Design review of the part built by this model. Coordinates are the model's own, in mm. A direction names the side the tool comes from. Give positions to 0.01 mm unless a question says otherwise; leave off trailing zeros. Write each loop counter-clockwise with the first axis right and the second up, starting at its lowest first coordinate (ties: lowest second). Pieces come first, ordered by that corner, then holes. Notation, with made-up numbers: M -13.75,-32 L -7.75,-32 A10 cw -7.75,-22 Z; hole C 85,56 d1. An arc over 180 degrees is marked long. Write each question's results on one line, items separated by ' | '. Start each with the question number.
from build123d import *

# Parameters (mm, degrees)
SKETCH1_W                       = 125
SKETCH1_H                       = 135
SKETCH1_W_2                     = 112.037037038
SKETCH1_H_2                     = 121
BOSS_EXTRUDE1_DEPTH             = 150
SKETCH3_W                       = 5
SKETCH3_H                       = 50
CUT_EXTRUDE1_DEPTH              = 68.5
CUT_EXTRUDE1_DEPTH_BACK         = 68.5
CUT_EXTRUDE2_REACH              = 127
SKETCH4_W                       = 60
SKETCH4_H                       = 40
CUT_EXTRUDE3_DEPTH              = 37.5
F_2_CLEARANCE_HOLE1_D           = 2.032
F_2_CLEARANCE_HOLE1_DEPTH       = 6.481481481
F_3_CLEARANCE_HOLE1_D           = 2.54
F_3_CLEARANCE_HOLE1_DEPTH       = 3.175
F_3_CLEARANCE_HOLE1_CSINK_D     = 3.9116
F_3_CLEARANCE_HOLE1_CSINK_ANGLE = 90
F_3_CLEARANCE_HOLE1_TIP         = 0.763092986
CUT_EXTRUDE4_REACH              = 122
SKETCH19_W                      = 121
SKETCH19_H                      = 50


with BuildPart() as part:
    # Sketch1 → Boss-Extrude1 (new body)
    with BuildSketch(Plane(origin=(0, 0, 0), x_dir=(1, 0, 0), z_dir=(0, 1, 0))):
        Rectangle(SKETCH1_W, SKETCH1_H)
        Rectangle(SKETCH1_W_2, SKETCH1_H_2, mode=Mode.SUBTRACT)
    extrude(amount=BOSS_EXTRUDE1_DEPTH)

    # Sketch3 → Cut-Extrude1 (cut, two sides)
    with BuildSketch(Plane.XY) as cut_extrude1_sk:
        with Locations((-60, 25)):
            Rectangle(SKETCH3_W, SKETCH3_H)
    extrude(amount=CUT_EXTRUDE1_DEPTH, mode=Mode.SUBTRACT)
    extrude(cut_extrude1_sk.sketch, amount=-CUT_EXTRUDE1_DEPTH_BACK, mode=Mode.SUBTRACT)

    # Sketch4 → Cut-Extrude2 (cut, up to next)
    with BuildSketch(Plane(origin=(62.5, 0, 0), x_dir=(0, 0, -1), z_dir=(1, 0, 0)), mode=Mode.PRIVATE) as cut_extrude2_sk1:
        with Locations((0, 20)):
            Rectangle(SKETCH4_W, SKETCH4_H)
    cut_extrude2_tool1 = extrude(cut_extrude2_sk1.sketch, amount=-CUT_EXTRUDE2_REACH, mode=Mode.PRIVATE) & part.part
    add(cut_extrude2_tool1.solids().sort_by_distance((62.5, 20, 0))[0], mode=Mode.SUBTRACT)

    # Sketch11 → #10 Clearance Hole1 (revolve, cut)
    with BuildSketch(Plane(origin=(-42.5, 15, 67.5), x_dir=(0, -1, 0), z_dir=(1, 0, 0))):
        Polygon((0, 0), (0, 26.849876674), (2.413, 25.4), (2.413, 0), align=None)
    f_10_clearance_hole1 = revolve(axis=Axis((-42.5, 15, 73.85), (0, 0, -1)), mode=Mode.SUBTRACT)

    # Mirror1: #10 Clearance Hole1 across plane
    add(f_10_clearance_hole1.mirror(Plane.XY), mode=Mode.SUBTRACT)

    # Sketch12 → Cut-Extrude3 (cut, symmetric)
    with BuildSketch(Plane.XY):
        with BuildLine():
            Line((56.018518519, 39), (56.018518519, 34))
            Line((56.018518519, 34), (59.259259259, 34))
            ThreePointArc((59.259259259, 34), (61.759259259, 36.5), (59.259259259, 39))
            Line((59.259259259, 39), (56.018518519, 39))
        make_face()
    extrude(amount=CUT_EXTRUDE3_DEPTH, both=True, mode=Mode.SUBTRACT)

    # #2 Clearance Hole1
    with Locations(Plane(origin=(62.5, 0, 0), x_dir=(0, 0, -1), z_dir=(1, 0, 0))):
        with Locations((-18.3915, 127.656921), (-18.3915, 82.156921)):
            Hole(F_2_CLEARANCE_HOLE1_D / 2, depth=F_2_CLEARANCE_HOLE1_DEPTH)

    # #3 Clearance Hole1
    with Locations(Plane(origin=(-56.018518519, 0, 0), x_dir=(0, 0, -1), z_dir=(1, 0, 0))):
        with Locations((10.2126, 67.112098568), (18.7126, 67.112098568)):
            CounterSinkHole(F_3_CLEARANCE_HOLE1_D / 2, F_3_CLEARANCE_HOLE1_CSINK_D / 2, depth=F_3_CLEARANCE_HOLE1_DEPTH, counter_sink_angle=F_3_CLEARANCE_HOLE1_CSINK_ANGLE)
            with Locations((0, 0, -(F_3_CLEARANCE_HOLE1_DEPTH + F_3_CLEARANCE_HOLE1_TIP / 2))):  # 118° drill point
                Cone(0, F_3_CLEARANCE_HOLE1_D / 2, F_3_CLEARANCE_HOLE1_TIP, mode=Mode.SUBTRACT)

    # Sketch19 → Cut-Extrude4 (cut, up to next)
    with BuildSketch(Plane.ZY.offset(57.5), mode=Mode.PRIVATE) as cut_extrude4_sk1:
        with Locations((0, 25)):
            Rectangle(SKETCH19_W, SKETCH19_H)
    cut_extrude4_tool1 = extrude(cut_extrude4_sk1.sketch, amount=-CUT_EXTRUDE4_REACH, mode=Mode.PRIVATE) & part.part
    add(cut_extrude4_tool1.solids().sort_by_distance((-57.5, 25, 0))[0], mode=Mode.SUBTRACT)


solid = part.part
Q1. We need section C-C on y = 15. Write out the cut boundary in (x, z), and give its area (3 significant figures).
Q2. We need section B-B on y = 36.5. Write out the cut boundary in (x, z), and give its area (3 significant figures).
Q3. For faces 4 (the flat face through (59, 20, -30)), 5 (the flat face through (59, 37, -37.5)), 6 (the flat face through (62.5, 74, 1)), 7 (the flat face through (-57.5, 25, -64)), list the 3-axis set-ups (+Z, -Z, +X, -X, +Y, -Y) from which the entire face can be reached by the end or side of a thin tool; tool diameter is ignored.
Q4. For pin 1 Ø3 at (x, z) = (60.5, 2.5) entering from -Y; pin 2 Ø7 at (x, z) = (-58.5, 13.5) entering from -Y; pin 3 Ø5.5 at (y, z) = (28, 64) entering from -X, all flat-tipped, find the tip position at first contact; note any pin that passes through.
Q5. We need section A-A on x = -35. Write out the cut boundary in (y, z), and give its area (3 significant figures).
Q6. The part is to be moulded in two halves that separate along X. For faces 1 (the cylindrical face through (61.76, 36.45, -33.7)), 2 (the flat face through (-56.019, 99, 1)), 3 (the flat face through (-1, 74, -67.5)), say which applies: pulls with the +X half, pulls with the -X half, needs draft (parallel to the pull), parting line crosses it, or undercut.
Q7. Wall thickness on line 1 along Y through (x, z) = (57, 18.5); line 2 along X through (y, z) = (63, 13.5); line 3 along X through (y, z) = (15, 63): over which ranges is each line inside the solid? List them lowest first. Write a range as from..to.
Q8. We need section D-D on z = 34.5. Write out the cut boundary in (x, y).
Answer sheet:
1) outline: M -57.5,-67.5 L -44.91,-67.5 L -44.91,-60.5 L -57.5,-60.5 Z; M -57.5,60.5 L -44.91,60.5 L -44.91,67.5 L -57.5,67.5 Z; M -40.09,-67.5 L 62.5,-67.5 L 62.5,-30 L 56.02,-30 L 56.02,-60.5 L -40.09,-60.5 Z; M -40.09,60.5 L 56.02,60.5 L 56.02,30 L 62.5,30 L 62.5,67.5 L -40.09,67.5 Z | area: 2,010 mm^2
2) outline: M -57.5,-67.5 L 62.5,-67.5 L 62.5,-30 L 61.76,-30 L 61.76,-37.5 L 56.02,-37.5 L 56.02,-60.5 L -57.5,-60.5 Z; M -57.5,60.5 L 56.02,60.5 L 56.02,37.5 L 61.76,37.5 L 61.76,30 L 62.5,30 L 62.5,67.5 L -57.5,67.5 Z | area: 1,990 mm^2
3) face 4: +X, -X, -Y | face 5: -X | face 6: +Z, -Z, +X, +Y, -Y | face 7: +Z, -Z, -X, -Y
4) pin 1: y = 40 | pin 2: y = 50 | pin 3: x = -57.5
5) outline: M 0,-67.5 L 150,-67.5 L 150,-60.5 L 0,-60.5 Z; M 0,60.5 L 150,60.5 L 150,67.5 L 0,67.5 Z | area: 2,100 mm^2
6) face 1: pulls with the -X half | face 2: undercut | face 3: needs draft
7) line 1: 40..81.15, 83.17..126.65, 128.67..150 | line 2: -62.5..-56.02, 56.02..62.5 | line 3: -57.5..-44.91, -40.09..62.5
8) outline: M -62.5,50 L -56.02,50 L -56.02,150 L -62.5,150 Z; M 56.02,0 L 62.5,0 L 62.5,150 L 56.02,150 L 56.02,39 L 59.26,39 A2.5 cw 59.26,34 L 56.02,34 Z
